```python
from build123d import *

# Parameters (mm, degrees)
SKETCH_1_R      = 26.7
EXTRUDE_1_DEPTH = 28.8
SKETCH_4_R      = 13
EXTRUDE_2_DEPTH = 39
CHAMFER_1_SIZE  = 1
CHAMFER_1_SIZE2 = 1.5


with BuildPart() as part:
    # Sketch 1 → Extrude 1 (new body)
    with BuildSketch(Plane(origin=(0, 0, 0), x_dir=(1, 0, 0), z_dir=(0, 1, 0))):
        with Locations(Location((0, 0, 0), (0, 0, 270))):
            Circle(SKETCH_1_R)
    extrude(amount=EXTRUDE_1_DEPTH)

    # Sketch 2 → Revolve 1 (revolve)
    with BuildSketch(Plane.XY, mode=Mode.PRIVATE) as revolve_1_sk:
        Polygon((-27.7, 28.8), (-26.7, 28.8), (0, 28.8), (0, 29), (-27.7, 29), align=None)
    revolve(revolve_1_sk.sketch.rotate(Axis((0, 37.25413602, 0), (0, -1, 0)), 270), axis=Axis((0, 37.25413602, 0), (0, -1, 0)))

    # Sketch 2_3 → Revolve 2 (revolve)
    with BuildSketch(Plane.XY, mode=Mode.PRIVATE) as revolve_2_sk:
        with BuildLine():
            ThreePointArc((-31.5, 32.8), (-28.812994231, 31.687005769), (-27.7, 29))
            Line((-27.7, 29), (0, 29))
            Line((0, 29), (0, 32.8))
            Line((0, 32.8), (-31.5, 32.8))
        make_face()
    revolve(revolve_2_sk.sketch.rotate(Axis((0, 37.25413602, 0), (0, -1, 0)), 270), axis=Axis((0, 37.25413602, 0), (0, -1, 0)))

    # Sketch 3 → Revolve 3 (revolve)
    with BuildSketch(Plane.XY, mode=Mode.PRIVATE) as revolve_3_sk:
        Polygon((-27.7, 0), (-26.7, 0), (0, 0), (0, -1.2), (-27.7, -1.2), align=None)
    revolve(revolve_3_sk.sketch.rotate(Axis((0, 9.532579507, 0), (0, -1, 0)), 270), axis=Axis((0, 9.532579507, 0), (0, -1, 0)))

    # Sketch 4 → Extrude 2 (add)
    with BuildSketch(Plane.XZ.offset(1.2)):
        with Locations(Location((0, 0, 0), (0, 0, 270))):
            Circle(SKETCH_4_R)
    extrude(amount=EXTRUDE_2_DEPTH)

    # Chamfer 1
    chamfer_1_edges = [part.edges().sort_by_distance(p)[0] for p in [
        (0, -40.2, 13),
    ]]
    chamfer_1_side = [part.faces().sort_by_distance(p)[0] for p in [
        (0, -20.7, 13),
    ]]
    chamfer(chamfer_1_edges, length=CHAMFER_1_SIZE, length2=CHAMFER_1_SIZE2, reference=chamfer_1_side[0])

    # Sketch 6 → Revolve 4 (revolve)
    with BuildSketch(Plane.XY, mode=Mode.PRIVATE) as revolve_4_sk:
        Polygon((-13, -1.2), (-13, -5.2), (-27.7, -1.2), align=None)
    revolve(revolve_4_sk.sketch.rotate(Axis((0, 5.765222619, 0), (0, -1, 0)), 270), axis=Axis((0, 5.765222619, 0), (0, -1, 0)))

    # Sketch 7 → Cut-Revolve 1 (revolve, cut)
    with BuildSketch(Plane.XY, mode=Mode.PRIVATE) as cut_revolve_1_sk:
        Polygon((-13, -5.2), (-12, -5.2), (-13, -7.2), align=None)
    revolve(cut_revolve_1_sk.sketch.rotate(Axis((0, -1.925824923, 0), (0, -1, 0)), 270), axis=Axis((0, -1.925824923, 0), (0, -1, 0)), mode=Mode.SUBTRACT)

    # Sketch 8 → Revolve 5 (revolve)
    with BuildSketch(Plane.XY, mode=Mode.PRIVATE) as revolve_5_sk:
        Polygon((0, 32.8), (0, 35.8), (-2, 35.8), (-4, 32.8), align=None)
    revolve(revolve_5_sk.sketch.rotate(Axis((0, 18.882882331, 0), (0, 1, 0)), 90), axis=Axis((0, 18.882882331, 0), (0, 1, 0)))


solid = part.part
```
Verification items for the finished model (mm, model axes). A direction names the side the tool comes from. Give positions to 0.01 mm unless a question says otherwise; leave off trailing zeros. Order: outer loops, then holes, each group sorted by start corner. A loop starts at its lowest first (then second) coordinate and runs counter-clockwise, first axis right, second up. Notation, with made-up numbers: (-11.5, 25.5) - (29.5, 25.5) arc R25 ccw to (29.5, 47.5) - close; hole circle Ø8 at (17, 46). An arc over 180 degrees is marked (long way). Answer as CSV lines item,"result". Start each with the question number.
Item 1: Material ranges on L1, parallel to Z at x = 0.5, y = 14; L2, parallel to Y at x = 5, z = -25; L3, parallel to Z at x = -16, y = 8.5, recorded low to high.
Item 2: Gauge pin test, flat ends, axial feed: pin 1 (3 mm diameter, centred on x = 15.5, y = -11.5, fed in from -Z); pin 2 (8 mm diameter, centred on x = 23, z = -14, fed in from -Y); pin 3 (19 mm diameter, centred on x = -2, z = 0.5, fed in from +Y); pin 4 (5 mm diameter, centred on x = 13.5, y = 20.5, fed in from +Z). Record the tip position at first contact, or that the pin passes through.
Item 3: Section check C-C, the plane y = -26.5. Record the boundary of the cut face in (x, z).
Item 4: Section check B-B, the plane x = 0. Record the boundary of the cut face in (y, z), plus the area to 3 significant figures.
Item 5: Access from +Z, -Z, +X, -X, +Y, -Y to the whole of each face (thin tool, end or side, straight path). Record for faces 1 (the face through (27.041, -0.592, -6.005)), 2 (the face through (0.093, 35.612, -2.123)), 3 (the face through (9, -5.2, 9)).
Item 6: Section check A-A, the plane z = 0. Record the boundary of the cut face in (x, y).
Item 7: Section check D-D, the plane y = 7.5. Record the boundary of the cut face in (x, z), plus the area to 3 significant figures.
Item 8: Mould release check, pull along Y, two halves, no side actions. Record for faces 4 (the face through (0, -40.2, 0)), 5 (the face through (0, 35.8, 0)), 6 (the face through (-7.91, -22.976, 10.316)), 7 (the face through (-14, 28.8, -23)): released by +Y, released by -Y, zero draft, split by the parting line, or undercut.
Filled in:
1,L1,"-26.7 to 26.7"
1,L2,"-1.8 to 32.8"
1,L3,"-21.37 to 21.37"
2,pin 1,"through"
2,pin 2,"y = -2.5"
2,pin 3,"y = 35.8"
2,pin 4,"z = 24.33"
3,outline,"circle Ø26 at (0, 0)"
4,outline,"(-40.2, -11.5) - (-39.2, -13) - (-7.2, -13) - (-5.2, -12) - (-5.2, -13) - (-1.2, -27.7) - (0, -27.7) - (0, -26.7) - (28.8, -26.7) - (28.8, -27.7) - (29, -27.7) arc R3.8 cw to (32.8, -31.5) - (32.8, -4) - (35.8, -2) - (35.8, 2) - (32.8, 4) - (32.8, 31.5) arc R3.8 cw to (29, 27.7) - (28.8, 27.7) - (28.8, 26.7) - (0, 26.7) - (0, 27.7) - (-1.2, 27.7) - (-5.2, 13) - (-5.2, 12) - (-7.2, 13) - (-39.2, 13) - (-40.2, 11.5) - close"
4,area,"2,920 mm^2"
5,face 1,"-Y"
5,face 2,"+Y"
5,face 3,"none"
6,outline,"(-31.5, 32.8) arc R3.8 cw to (-27.7, 29) - (-27.7, 28.8) - (-26.7, 28.8) - (-26.7, 0) - (-27.7, 0) - (-27.7, -1.2) - (-13, -5.2) - (-12, -5.2) - (-13, -7.2) - (-13, -39.2) - (-11.5, -40.2) - (11.5, -40.2) - (13, -39.2) - (13, -7.2) - (12, -5.2) - (13, -5.2) - (27.7, -1.2) - (27.7, 0) - (26.7, 0) - (26.7, 28.8) - (27.7, 28.8) - (27.7, 29) arc R3.8 cw to (31.5, 32.8) - (4, 32.8) - (2, 35.8) - (-2, 35.8) - (-4, 32.8) - close"
7,outline,"circle Ø53.4 at (0, 0)"
7,area,"2,240 mm^2"
8,face 4,"released by -Y"
8,face 5,"released by +Y"
8,face 6,"zero draft"
8,face 7,"undercut"
